from build123d import *

# Parameters (mm, degrees)
PAD_DEPTH          = 2
SKETCH001_R        = 1.8
SKETCH001_W        = 4
SKETCH001_H        = 16
POCKET_DEPTH       = 2.001
SKETCH002_R        = 2
POCKET001_DEPTH    = 2.001
SKETCH003_W        = 17
SKETCH003_H        = 43.9
POCKET002_DEPTH    = 2.001
SKETCH004_R        = 2
POCKET003_DEPTH    = 2.001
POCKET011002_DEPTH = 2.001


with BuildPart() as part:
    # Sketch → Pad (new body)
    with BuildSketch(Plane.XY):
        with BuildLine():
            Line((65.081198, 28.5), (-65.081198, 28.5))
            Line((-65.081198, 28.5), (-69.7, 36.5))
            Line((-69.7, 36.5), (-79, 36.5))
            ThreePointArc((-79, 36.5), (-81.828427, 35.328427), (-83, 32.5))
            Line((-83, 32.5), (-83, 9.254741))
            Line((-83, 9.254741), (-70, -28.5))
            Line((-42.5, -28.5), (-70, -28.5))
            Line((-42.5, -28.5), (-38.5, -32.5))
            Line((-38.5, -32.5), (38.5, -32.5))
            Line((38.5, -32.5), (42.5, -28.5))
            Line((42.5, -28.5), (70, -28.5))
            Line((70, -28.5), (83, 9.254741))
            Line((83, 9.254741), (83, 32.5))
            ThreePointArc((83, 32.5), (81.828427, 35.328427), (79, 36.5))
            Line((79, 36.5), (69.7, 36.5))
            Line((69.7, 36.5), (65.081198, 28.5))
        make_face()
    extrude(amount=-PAD_DEPTH)

    # Sketch001 → Pocket (cut, through all)
    with BuildSketch(Plane.XY):
        with Locations((-79, 29.5)):
            Circle(SKETCH001_R)
        with Locations((-79, 13)):
            Circle(SKETCH001_R)
        with Locations((79, 29.5)):
            Circle(SKETCH001_R)
        with Locations((79, 13)):
            Circle(SKETCH001_R)
        with Locations((-72, 21.25)):
            Rectangle(SKETCH001_W, SKETCH001_H)
        with Locations((72, 21.25)):
            Rectangle(SKETCH001_W, SKETCH001_H)
    extrude(amount=-POCKET_DEPTH, mode=Mode.SUBTRACT)

    # Sketch002 → Pocket001 (cut, through all)
    with BuildSketch(Plane.XY):
        with Locations((-16.5, -12.5)):
            Circle(SKETCH002_R)
        with Locations((35, -12.5)):
            Circle(SKETCH002_R)
        with BuildLine():
            Line((-33.5, -4), (-20.5, -4))
            Line((-20.5, -4), (-20.5, -18.5))
            Line((-20.5, -18.5), (-18.5, -18.5))
            Line((-18.5, -18.5), (-18.5, -26.5))
            Line((-18.5, -26.5), (-26.171714, -26.5))
            ThreePointArc((-29.028286, -26.5), (-27.6, -29.9), (-26.171714, -26.5))
            Line((-33.5, -26.5), (-29.028286, -26.5))
            Line((-33.5, -26.5), (-33.5, -4))
        make_face()
        with BuildLine():
            Line((18, -4), (31, -4))
            Line((31, -4), (31, -18.5))
            Line((31, -18.5), (33, -18.5))
            Line((33, -18.5), (33, -26.5))
            Line((25.228286, -26.5), (33, -26.5))
            ThreePointArc((22.371714, -26.5), (23.8, -29.9), (25.228286, -26.5))
            Line((22.371714, -26.5), (18, -26.5))
            Line((18, -26.5), (18, -4))
        make_face()
    extrude(amount=-POCKET001_DEPTH, mode=Mode.SUBTRACT)

    # Sketch003 → Pocket002 (cut, through all)
    with BuildSketch(Plane.XY):
        Polygon((-59.5, 12.4), (-42.5, 12.4), (-42.5, -28.5), (-42.5, -31.5), (-59.5, -31.5), (-59.5, -28.5), align=None)
        with Locations((51, -9.55)):
            Rectangle(SKETCH003_W, SKETCH003_H)
    extrude(amount=-POCKET002_DEPTH, mode=Mode.SUBTRACT)

    # Sketch004 → Pocket003 (cut, through all)
    with BuildSketch(Plane.XY):
        with Locations((-8.5, 23.5)):
            Circle(SKETCH004_R)
        with Locations((8.5, 23.5)):
            Circle(SKETCH004_R)
    extrude(amount=-POCKET003_DEPTH, mode=Mode.SUBTRACT)

    # Sketch016 → Pocket011002 (cut, through all)
    with BuildSketch(Plane.XY):
        with BuildLine():
            Line((-1.5, 0), (1.5, 0))
            ThreePointArc((2.5, -1), (2.207107, -0.292893), (1.5, 0))
            Line((2.5, -1), (2.5, -11))
            ThreePointArc((1.5, -12), (2.207107, -11.707107), (2.5, -11))
            Line((1.5, -12), (-1.5, -12))
            ThreePointArc((-2.5, -11), (-2.207107, -11.707107), (-1.5, -12))
            Line((-2.5, -11), (-2.5, -1))
            ThreePointArc((-1.5, 0), (-2.207107, -0.292893), (-2.5, -1))
        make_face()
    extrude(amount=-POCKET011002_DEPTH, mode=Mode.SUBTRACT)


solid = part.part
Check sheet for the modelled part. Datum: model origin and axes. Units: mm. A direction names the side the tool comes from. Coordinates: 2 decimals unless noted, no trailing zeros. Loops run counter-clockwise (first coordinate to the right, second up) from the corner with the lowest first, then second, coordinate; pieces in that order, holes last. Notation, with made-up numbers: (64, 13.5) -> (106, 13.5) arc R15 cw to (106, 35.5) -> close; hole circle Ø8 at (54.5, 63.25). An arc over 180 degrees is marked (long way). Answer in a Markdown table with one row per item.
1. Go/stop test with flat-tipped pins: pin 1 (5 mm diameter, centred on x = -27.6, y = -27.9, fed in from -Z); pin 2 (0.6 mm diameter, centred on y = -8, z = -1.5, fed in from -X); pin 3 (0.6 mm diameter, centred on y = -13.5, z = -1, fed in from -X); pin 4 (0.6 mm diameter, centred on x = -31.5, z = -1, fed in from +Y). Record where each tip stops, or that it passes through.
Check values:
| item | result |
|---|---|
| pin 1 | stops at z = -2 |
| pin 2 | stops at x = -77.16 |
| pin 3 | stops at x = -75.27 |
| pin 4 | stops at y = 28.5 |
2. Release check for a two-part mould opening along X. For faces 1 (the face through (76.41, -9.89, -0.99)), 2 (the face through (-1, 2, -2)), 3 (the face through (-80.327, 14.217, -0.986)) record: released by +X, released by -X, zero draft, split by the parting line, or undercut.
Check values:
| item | result |
|---|---|
| face 1 | released by +X |
| face 2 | zero draft |
| face 3 | undercut |
3. Sectioned sample at C-C, the plane x = -32. Record the boundary of the cut face in (y, z).
Check values:
| item | result |
|---|---|
| outline | (-32.5, -2) -> (-26.5, -2) -> (-26.5, 0) -> (-32.5, 0) -> close; (-4, -2) -> (28.5, -2) -> (28.5, 0) -> (-4, 0) -> close |
4. Access from +Z, -Z, +X, -X, +Y, -Y to the whole of each face (thin tool, end or side, straight path). Record for faces 4 (the face through (67.423, 32.556, -0.986)), 5 (the face through (-17.974, -11.148, -0.986)).
Check values:
| item | result |
|---|---|
| face 4 | +Z, -Z, +Y |
| face 5 | +Z, -Z |
5. Material ranges on line 1 along X through (y, z) = (18.5, -0.8); line 2 along Y through (x, z) = (8.5, -0.6); line 3 along X through (y, z) = (-16, -0.55), recorded low to high. Write a range as [from, to].
Check values:
| item | result |
|---|---|
| line 1 | x = [-83, -74], [-70, 70], [74, 83] |
| line 2 | y = [-32.5, 21.5], [25.5, 28.5] |
| line 3 | x = [-74.3, -59.5], [-42.5, -33.5], [-20.5, 18], [31, 42.5], [59.5, 74.3] |
6. Sectioned sample at D-D, the plane y = 2. Record the boundary of the cut face in (x, z).
Check values:
| item | result |
|---|---|
| outline | (-80.5, -2) -> (-59.5, -2) -> (-59.5, 0) -> (-80.5, 0) -> close; (-42.5, -2) -> (42.5, -2) -> (42.5, 0) -> (-42.5, 0) -> close; (59.5, -2) -> (80.5, -2) -> (80.5, 0) -> (59.5, 0) -> close |
7. Sectioned sample at A-A, the plane y = 23.5. Record the boundary of the cut face in (x, z), then the cut area to 3 significant figures.
Check values:
| item | result |
|---|---|
| outline | (-83, -2) -> (-74, -2) -> (-74, 0) -> (-83, 0) -> close; (-70, -2) -> (-10.5, -2) -> (-10.5, 0) -> (-70, 0) -> close; (-6.5, -2) -> (6.5, -2) -> (6.5, 0) -> (-6.5, 0) -> close; (10.5, -2) -> (70, -2) -> (70, 0) -> (10.5, 0) -> close; (74, -2) -> (83, -2) -> (83, 0) -> (74, 0) -> close |
| area | 300 mm2 |
8. Sectioned sample at B-B, the plane x = -8.5. Record the boundary of the cut face in (y, z), then the cut area to 3 significant figures.
Check values:
| item | result |
|---|---|
| outline | (-32.5, -2) -> (21.5, -2) -> (21.5, 0) -> (-32.5, 0) -> close; (25.5, -2) -> (28.5, -2) -> (28.5, 0) -> (25.5, 0) -> close |
| area | 114 mm2 |
